from build123d import *

# Parameters (mm, degrees)
SKETCH1_R                   = 29.5
BOSS_EXTRUDE1_DEPTH         = 12.7
SKETCH2_R                   = 19
BOSS_EXTRUDE2_DEPTH         = 1.905
F_3_4_0_75_DIAMETER_HOLE1_D = 19.05
CUT_EXTRUDE1_DEPTH          = 44.60951731
CUT_EXTRUDE1_DEPTH_BACK     = 44.60951731
SKETCH7_R                   = 2
SKETCH8_W                   = 4.7625
SKETCH8_H                   = 4.7625
CUT_EXTRUDE2_DEPTH          = 45.201878071


with BuildPart() as part:
    # Sketch1 → Boss-Extrude1 (new body)
    with BuildSketch(Plane(origin=(0, 0, 0), x_dir=(1, 0, 0), z_dir=(0, 1, 0))):
        with Locations(Location((0, 0, 0), (0, 0, 270))):
            Circle(SKETCH1_R)
    extrude(amount=BOSS_EXTRUDE1_DEPTH)

    # Sketch2 → Boss-Extrude2 (add)
    with BuildSketch(Plane(origin=(0, 12.7, 0), x_dir=(1, 0, 0), z_dir=(0, 1, 0))):
        with Locations(Location((0, 0, 0), (0, 0, 90))):
            Circle(SKETCH2_R)
    extrude(amount=BOSS_EXTRUDE2_DEPTH)

    # 3/4 (0.75) Diameter Hole1 (through all)
    with Locations(Plane(origin=(0.010328694, 14.605, -0.138454069), x_dir=(0, 0, 1), z_dir=(0, 1, 0))):
        with Locations((0, 0)):
            Hole(F_3_4_0_75_DIAMETER_HOLE1_D / 2)

    # Sketch7 → Cut-Extrude1 (cut, two sides: drawn at the far end of the back side and taken through both)
    with BuildSketch(Plane(origin=(0, 12.7, 0), x_dir=(1, 0, 0), z_dir=(0, 1, 0)).offset(-CUT_EXTRUDE1_DEPTH_BACK)):
        with Locations(Location((0, 25, 0), (0, 0, 270))):
            Circle(SKETCH7_R)
        with Locations(Location((21.650635095, 12.5, 0), (0, 0, 270))):
            Circle(SKETCH7_R)
        with Locations(Location((21.650635095, -12.5, 0), (0, 0, 270))):
            Circle(SKETCH7_R)
        with Locations(Location((0, -25, 0), (0, 0, 270))):
            Circle(SKETCH7_R)
        with Locations(Location((-21.650635095, -12.5, 0), (0, 0, 270))):
            Circle(SKETCH7_R)
        with Locations(Location((-21.650635095, 12.5, 0), (0, 0, 270))):
            Circle(SKETCH7_R)
    extrude(amount=CUT_EXTRUDE1_DEPTH + CUT_EXTRUDE1_DEPTH_BACK, mode=Mode.SUBTRACT)

    # Sketch8 → Cut-Extrude2 (cut, through all)
    with BuildSketch(Plane(origin=(0, 14.605, 0), x_dir=(1, 0, 0), z_dir=(0, 1, 0))):
        with Locations((0, 9.94446313)):
            Rectangle(SKETCH8_W, SKETCH8_H)
    extrude(amount=-CUT_EXTRUDE2_DEPTH, mode=Mode.SUBTRACT)


solid = part.part
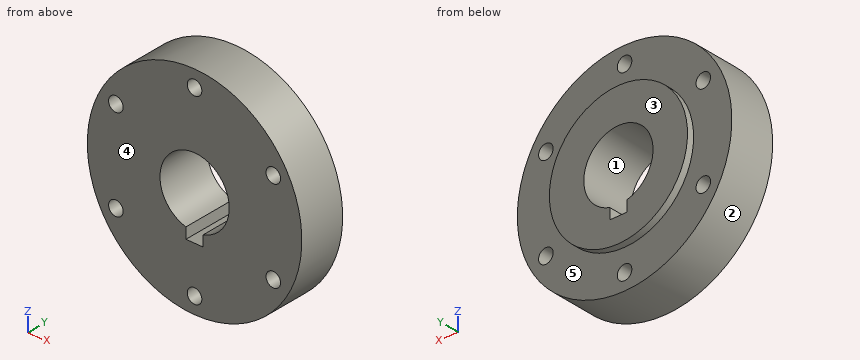
Work out the finished part from the listing and answer in its coordinate system (mm). Face numbers are marked on the shaded views. A direction names the side the tool comes from. Give positions to 0.01 mm unless a question says otherwise; leave off trailing zeros. Loops run counter-clockwise (first coordinate to the right, second up) from the corner with the lowest first, then second, coordinate; pieces in that order, holes last. Notation, with made-up numbers: (-16, 19) - (24, 19) arc R27 cw to (24, 50) - close; hole circle Ø6 at (79.25, 37). An arc over 180 degrees is marked (long way). Answer in a Markdown table with one row per item. Add a question column.
Q1. The part is cut by section A-A (x = 0). Determine the outline of the cut face in (y, z) (3 decimals), and give its area (3 significant figures).
Q2. A tool of negligible diameter and unlimited length cuts with its end or side. For the marked faces 4 and 5, from which of +Z, -Z, +X, -X, +Y, -Y can it reach the whole face along a straight path? Write none if from no direction.
Q3. The part is cut by section B-B (z = -25). Determine the outline of the cut face in (x, y), and give its area (3 significant figures).
Q4. Consider line 1 along X through (y, z) = (10, -12.5); line 2 along Z through (x, y) = (1, 5.75) (3 decimals); line 3 along X through (y, z) = (13, -1.5). Determine where each line is inside the solid, lowest interval first.
Q5. Each of these flat-tipped pins is pushed along its axis until it touches: P1, Ø2.5, axis at y = 5.5, z = -11.5, coming from the +X side; P2, Ø12, axis at x = -23.5, z = 10.5, coming from the +Y side; P3, Ø5, axis at y = 12, z = -22, coming from the -X side; P4, Ø3.5, axis at x = 0, z = -25, coming from the -Y side. Where does it stop, or does it pass through?
Q6. The part is cut by section C-C (z = 12.5). Determine the outline of the cut face in (x, y) (3 decimals), and give its area (3 significant figures).
Q7. The part is cut by section D-D (y = 13.5). Determine the outline of the cut face in (x, z) (3 decimals), and give its area (3 significant figures).
Q8. Determine the mould class of the marked faces 1, 2 and 3 for opening direction Z: released by +Z, released by -Z, zero draft, split by the parting line, or undercut.
Solution:
| question | item | result |
|---|---|---|
| 1 | outline | (0, -29.5) - (12.7, -29.5) - (12.7, -27) - (0, -27) - close; (0, -23) - (12.7, -23) - (12.7, -19) - (14.605, -19) - (14.605, -12.326) - (0, -12.326) - close; (0, 9.387) - (14.605, 9.387) - (14.605, 19) - (12.7, 19) - (12.7, 23) - (0, 23) - close; (0, 27) - (12.7, 27) - (12.7, 29.5) - (0, 29.5) - close |
| 1 | area | 403 mm² |
| 2 | face 4 | +Z, -Z, +X, -X, -Y |
| 2 | face 5 | +Y |
| 3 | outline | (-15.66, 0) - (-2, 0) - (-2, 12.7) - (-15.66, 12.7) - close; (2, 0) - (15.66, 0) - (15.66, 12.7) - (2, 12.7) - close |
| 3 | area | 347 mm² |
| 4 | line 1 | x = -26.72 to -23.65, -19.65 to 19.65, 23.65 to 26.72 |
| 4 | line 2 | z = -29.483 to -26.732, -23.268 to -12.326, 9.335 to 23.268, 26.732 to 29.483 |
| 4 | line 3 | x = -18.94 to -9.42, 9.44 to 18.94 |
| 5 | P1 | stops at x = 27.66 |
| 5 | P2 | stops at y = 12.7 |
| 5 | P3 | stops at x = -22.14 |
| 5 | P4 | passes through |
| 6 | outline | (-26.721, 0) - (-23.651, 0) - (-23.651, 12.7) - (-26.721, 12.7) - close; (-19.651, 0) - (19.651, 0) - (19.651, 12.7) - (14.309, 12.7) - (14.309, 14.605) - (-14.309, 14.605) - (-14.309, 12.7) - (-19.651, 12.7) - close; (23.651, 0) - (26.721, 0) - (26.721, 12.7) - (23.651, 12.7) - close |
| 6 | area | 632 mm² |
| 7 | outline | circle Ø38 at (0, 0); hole (-2.381, -12.326) - (2.381, -12.326) - (2.381, -9.364) arc R9.525 ccw (long way) to (-2.381, -9.358) - close |
| 7 | area | 836 mm² |
| 8 | face 1 | undercut |
| 8 | face 2 | split by the parting line |
| 8 | face 3 | zero draft |
